Verification items for the finished model (mm, model axes). A direction names the side the tool comes from. Coordinates: 2 decimals unless noted, no trailing zeros. Write each loop counter-clockwise with the first axis right and the second up, starting at its lowest first coordinate (ties: lowest second). Pieces come first, ordered by that corner, then holes. Notation, with made-up numbers: (42.5, 26.5) -> (84.5, 26.5) arc R15 ccw to (84.5, 48.5) -> close; hole circle Ø2 at (74, 49). An arc over 180 degrees is marked (long way). Answer in a Markdown table with one row per item.
```python
from build123d import *

# Parameters (mm, degrees)
F0_R     = 10
F1_DEPTH = 2


with BuildPart() as f1:
    # F0 (on Front) → F1 (new body)
    with BuildSketch(Plane.XZ):
        Circle(F0_R)
        Polygon((3.692769, 6.431684), (7.258024, -1.524532), (0.792936, -7.373897), (-6.767962, -3.032787), (-4.975767, 5.499532), align=None, mode=Mode.SUBTRACT)
    extrude(amount=F1_DEPTH)


solid = f1.part
```
1. Release check for a two-part mould opening along X. For faces 1 (the face through (-0.7, -0.99, 5.96)), 2 (the face through (7, -2, 0)), 3 (the face through (-2.17, -0.99, -9.76)), 4 (the face through (-5.884, -0.986, 1.174)) record: released by +X, released by -X, zero draft, split by the parting line, or undercut.
Findings below:
| item | result |
|---|---|
| face 1 | undercut |
| face 2 | zero draft |
| face 3 | split by the parting line |
| face 4 | undercut |
2. Access from +Z, -Z, +X, -X, +Y, -Y to the whole of each face (thin tool, end or side, straight path). Record for faces 5 (the face through (4.07, -0.99, -4.41)), 6 (the face through (7, 0, 0)).
Findings below:
| item | result |
|---|---|
| face 5 | +Y, -Y |
| face 6 | +Z, -Z, +X, -X, +Y |
3. Sectioned sample at A-A, the plane y = -0.7. Record the cut outline in (x, z), and give its area (3 significant figures).
Findings below:
| item | result |
|---|---|
| outline | circle Ø20 at (0, 0); hole (-6.77, -3.03) -> (0.79, -7.37) -> (7.26, -1.52) -> (3.69, 6.43) -> (-4.98, 5.5) -> close |
| area | 183 mm² |
4. Material ranges on probe 1 along Z at (x, y) = (-3, -0.4); probe 2 along Z at (x, y) = (1, -1.1); probe 3 along X at (y, z) = (-1.3, -2.25), recorded low to high. Write a range as from..to.
Findings below:
| item | result |
|---|---|
| probe 1 | z = -9.54..-5.2, 5.71..9.54 |
| probe 2 | z = -9.95..-7.19, 6.14..9.95 |
| probe 3 | x = -9.74..-6.6, 6.46..9.74 |
5. Sectioned sample at B-B, the plane z = 6. Record the cut outline in (x, y).
Findings below:
| item | result |
|---|---|
| outline | (-8, -2) -> (-0.32, -2) -> (-0.32, 0) -> (-8, 0) -> close; (3.89, -2) -> (8, -2) -> (8, 0) -> (3.89, 0) -> close |
6. Sectioned sample at C-C, the plane x = -2.5. Record the cut outline in (y, z).
Findings below:
| item | result |
|---|---|
| outline | (-2, -9.68) -> (0, -9.68) -> (0, -5.48) -> (-2, -5.48) -> close; (-2, 5.77) -> (0, 5.77) -> (0, 9.68) -> (-2, 9.68) -> close |
